Work out the finished part from the listing and answer in its coordinate system (mm). A direction names the side the tool comes from. Coordinates: 2 decimals unless noted, no trailing zeros. Answer as CSV lines item,"result".
```python
from build123d import *

# Parameters (mm, degrees)
CUT_EXTRUDE9_DEPTH  = 45.0000001
CUT_EXTRUDE10_REACH = 36.558
SKETCH8_R           = 1.5


with BuildPart() as part:
    # Sketch1 → Revolve1 (revolve)
    with BuildSketch(Plane(origin=(0, 0, 0), x_dir=(1, 0, 0), z_dir=(0, 1, 0))):
        with BuildLine():
            Line((0, 12), (0, 10.75))
            Line((0, 10.75), (3.5, 10.75))
            Line((3.5, 10.75), (18.5, 10.75))
            Line((18.5, 10.75), (20.5, 10.75))
            Line((20.5, 10.75), (24.5, 8.5))
            Line((24.5, 8.5), (26.5, 8.5))
            Line((26.5, 8.5), (26.5, 5.25))
            Line((26.5, 5.25), (42.375, 5.25))
            ThreePointArc((42.375, 5.25), (43.524048519, 8.024048519), (40.75, 6.875))
            Line((40.75, 6.875), (32.216506351, 6.875))
            ThreePointArc((32.216506351, 6.875), (30.922411125, 7.045370869), (29.716506351, 7.544872981))
            Line((29.716506351, 7.544872981), (28.062177826, 8.5))
            Line((28.062177826, 8.5), (22, 12))
            Line((22, 12), (0, 12))
        make_face()
    revolve(axis=Axis((-40.558590026, 0, 0), (1, 0, 0)))

    # Sketch5 → Revolve2 (revolve)
    with BuildSketch(Plane.XY):
        Polygon((22, -12), (15.07179677, -16), (2.309401077, -16), (0, -12), align=None)
    revolve(axis=Axis((-0.804180618, 0, 0), (1, 0, 0)))

    # Sketch7 → Cut-Extrude9 (cut, through all)
    with BuildSketch(Plane(origin=(0, 0, 0), x_dir=(0, 0, -1), z_dir=(1, 0, 0))):
        with BuildLine():
            ThreePointArc((1.25, 15.951097141), (0, 16), (-1.25, 15.951097141))
            Line((-1.25, 15.951097141), (1.25, 15.951097141))
        make_face()
        with BuildLine():
            Line((-11.832293992, -1.999204566), (-15.951097141, -1.25))
            ThreePointArc((-15.951097141, -1.25), (-11.313708499, -11.313708499), (-1.25, -15.951097141))
            Line((-1.25, -15.951097141), (-2, -11.832159566))
            ThreePointArc((-2, -11.832159566), (-8.485566586, -8.484996153), (-11.832293992, -1.999204566))
        make_face()
        with BuildLine():
            ThreePointArc((15.951097141, 1.25), (11.313708499, 11.313708499), (1.25, 15.951097141))
            Line((1.25, 15.951097141), (2, 11.832159566))
            ThreePointArc((2, 11.832159566), (8.485566586, 8.484996153), (11.832293992, 1.999204566))
            Line((11.832293992, 1.999204566), (15.951097141, 1.25))
        make_face()
        with BuildLine():
            Line((-15.951097141, 1.25), (-11.832159566, 2))
            ThreePointArc((-11.832159566, 2), (-8.484996153, 8.485566586), (-1.999204566, 11.832293992))
            Line((-1.999204566, 11.832293992), (-1.25, 15.951097141))
            ThreePointArc((-1.25, 15.951097141), (-11.313708499, 11.313708499), (-15.951097141, 1.25))
        make_face()
        with BuildLine():
            Line((1.999204566, -11.832293992), (1.25, -15.951097141))
            ThreePointArc((1.25, -15.951097141), (11.313708499, -11.313708499), (15.951097141, -1.25))
            Line((15.951097141, -1.25), (11.832159566, -2))
            ThreePointArc((11.832159566, -2), (8.484996153, -8.485566586), (1.999204566, -11.832293992))
        make_face()
        with BuildLine():
            Line((1.25, -15.951097141), (-1.25, -15.951097141))
            ThreePointArc((-1.25, -15.951097141), (0, -16), (1.25, -15.951097141))
        make_face()
        with BuildLine():
            Line((-15.951097141, -1.25), (-15.951097141, 1.25))
            ThreePointArc((-15.951097141, 1.25), (-16, 0), (-15.951097141, -1.25))
        make_face()
        with BuildLine():
            ThreePointArc((16, 0), (15.987769611, 0.625478115), (15.951097141, 1.25))
            Line((15.951097141, 1.25), (15.951097141, -1.25))
            ThreePointArc((15.951097141, -1.25), (15.987769611, -0.625478115), (16, 0))
        make_face()
    extrude(amount=CUT_EXTRUDE9_DEPTH, mode=Mode.SUBTRACT)

    # Sketch8 → Cut-Extrude10 (cut, up to next)
    with BuildSketch(Plane(origin=(0, -8.485281374, -8.485281374), x_dir=(1, 0, 0), z_dir=(0, 0.707106781, 0.707106781)), mode=Mode.PRIVATE) as cut_extrude10_sk1:
        with Locations((6, 0)):
            Circle(SKETCH8_R)
    cut_extrude10_tool1 = extrude(cut_extrude10_sk1.sketch, amount=CUT_EXTRUDE10_REACH, mode=Mode.PRIVATE) & part.part
    add(cut_extrude10_tool1.solids().sort_by_distance((6, -8.485281, -8.485281))[0], mode=Mode.SUBTRACT)


solid = part.part
```
(1) Which of the six approach directions +Z, -Z, +X, -X, +Y, -Y give full straight-line access (tool end or side, diameter ignored) to faces 1 (the face through (10.85, -13.92, 1.62)), 2 (the face through (25.514, 7.167, -4.57))?
Computed values:
face 1,"+Z, +X, -X, -Y"
face 2,"-X"
(2) For a pull along Z with two mould halves and no side action, classify faces 3 (the face through (10.39, 10.66, 1.4)), 4 (the face through (10.85, -13.86, -1.63)), 5 (the face through (34.5, 1.6, -5)), 6 (the face through (9, 0, 15.951)) as pulls with the +Z half, pulls with the -Z half, needs draft (parallel to the pull), parting line crosses it, or undercut.
Computed values:
face 3,"undercut"
face 4,"pulls with the -Z half"
face 5,"undercut"
face 6,"pulls with the +Z half"
(3) Flat-ended cylindrical pins translate along their axes: pin 1 Ø8 at (x, y) = (21, 1) entering from +Z; pin 2 Ø13.5 at (y, z) = (0, 0) entering from -X; pin 3 Ø10 at (y, z) = (0, 0) entering from +X; pin 4 Ø3 at (x, y) = (24.5, 0) entering from +Z. Find the tip coordinate at first contact, or state that the pin passes through.
Computed values:
pin 1,"z = 14.86"
pin 2,"x = 26.5"
pin 3,"through"
pin 4,"z = 11.42"
(4) Consider line 1 along Y through (x, z) = (12.5, 0); line 2 along Y through (x, z) = (37.75, 0) (3 decimals); line 3 along Z through (x, y) = (5, 5.5). Determine where each line is inside the solid, lowest interval first.
Computed values:
line 1,"-15.95 to -10.75, 10.75 to 15.95"
line 2,"-6.875 to -5.25, 5.25 to 6.875"
line 3,"-10.67 to -9.24, 9.24 to 10.67"
